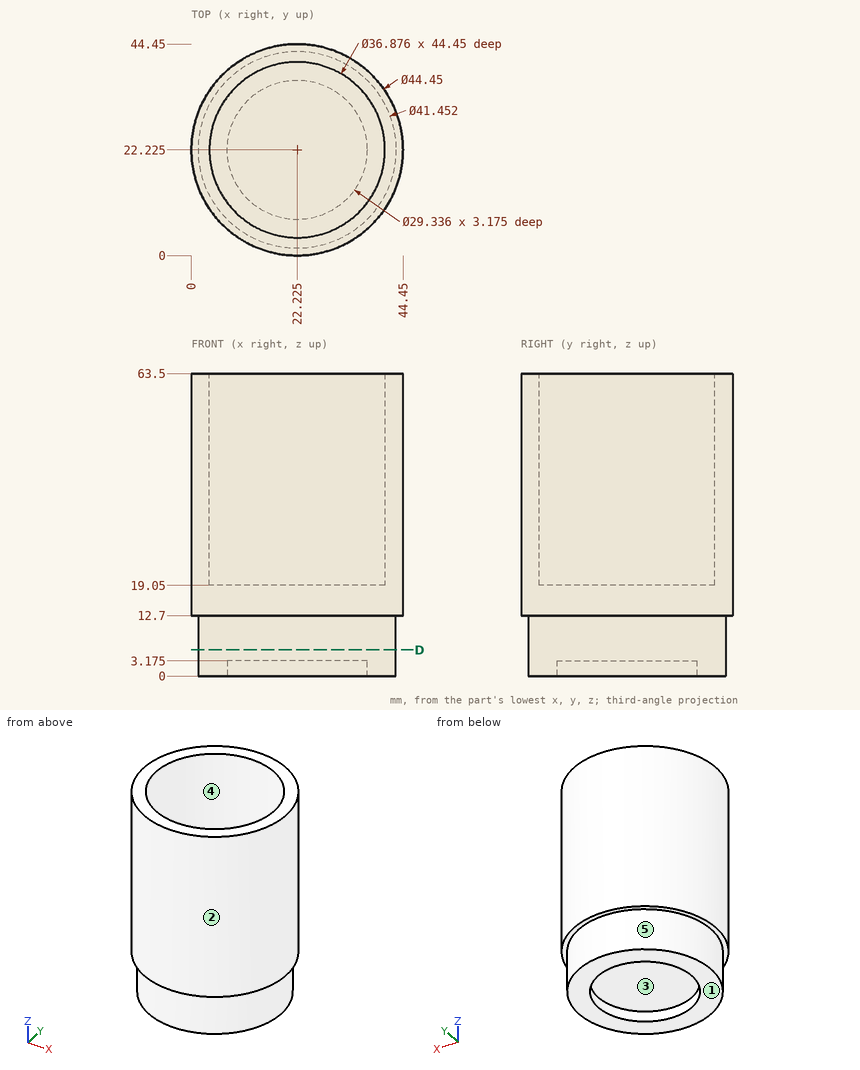
Drawing for the job (mm, zero at the part's lowest x, y, z). A direction names the side the tool comes from. Round coordinates to 2 decimals unless told otherwise and drop trailing zeros. Loops run counter-clockwise (first coordinate to the right, second up) from the corner with the lowest first, then second, coordinate; pieces in that order, holes last.
1. Wall check: probe 1 along X at (y, z) = (21.5, 61); probe 2 along Z at (x, y) = (28.5, 7); probe 3 along X at (y, z) = (38, 45.5). Give the ranges that are in metal, low to high.
Check values:
probe 1: x = 0.01 to 3.8, 40.65 to 44.44
probe 2: z = 0 to 19.05
probe 3: x = 6.57 to 12.68, 31.77 to 37.88
2. Mould opens along Y. For the marked faces 1, 2 and 3 say: +Y half, -Y half, draft (parallel to the pull), parting line (faces both ways), or undercut.
Check values:
face 1: draft
face 2: parting line
face 3: undercut
3. Band-saw the part on D-D, the plane z = 5.5. List the corners of the cut face in (x, y) (1 decimal), and give its area (3 significant figures).
Check values:
outline: circle Ø41.5 at (22.2, 22.2)
area: 1,350 mm2
4. Tool access for the marked faces 4 and 5: list every direction of +Z, -Z, +X, -X, +Y, -Y with a clear straight run to the whole face (end or side of a thin tool).
Check values:
face 4: +Z
face 5: -Z
5. Drop flat-ended pins along their axis: P1, Ø3, axis at x = 37.5, y = 29.5, coming from the -Z side; P2, Ø8, axis at x = 23.5, z = 40, coming from the +Y side; P3, Ø3, axis at x = 31, y = 28.5, coming from the +Z side; P4, Ø3, axis at y = 30, z = 40.5, coming from the +X side. Give the stop position or say it passes through.
Check values:
P1: stops at z = 0
P2: stops at y = 44.45
P3: stops at z = 19.05
P4: stops at x = 43.55
